```python
from build123d import *

# Parameters (mm, degrees)
SKETCH2_W           = 127
SKETCH2_H           = 70
BOSS_EXTRUDE1_DEPTH = 55
SKETCH4_W           = 127
SKETCH4_H           = 30
CUT_EXTRUDE1_DEPTH  = 50
SKETCH5_W           = 15
SKETCH5_H           = 23
BOSS_EXTRUDE2_DEPTH = 23
SKETCH6_W           = 3
SKETCH6_H           = 23
CUT_EXTRUDE2_DEPTH  = 23
SKETCH9_W           = 15
SKETCH9_H           = 10
CUT_EXTRUDE3_DEPTH  = 11.5
SKETCH10_W          = 117
SKETCH10_H          = 60
CUT_EXTRUDE4_DEPTH  = 1
SKETCH12_R          = 5
CUT_EXTRUDE5_DEPTH  = 300


with BuildPart() as part:
    # Sketch2 → Boss-Extrude1 (new body)
    with BuildSketch(Plane(origin=(0, 0, 0), x_dir=(1, 0, 0), z_dir=(0, 1, 0))):
        Rectangle(SKETCH2_W, SKETCH2_H)
    extrude(amount=BOSS_EXTRUDE1_DEPTH)

    # Sketch4 → Cut-Extrude1 (cut)
    with BuildSketch(Plane(origin=(0, 0, 0), x_dir=(1, 0, 0), z_dir=(0, 1, 0))):
        Rectangle(SKETCH4_W, SKETCH4_H)
    extrude(amount=CUT_EXTRUDE1_DEPTH, mode=Mode.SUBTRACT)

    # Sketch5 → Boss-Extrude2 (add)
    with BuildSketch(Plane.XZ.offset(-50)):
        Rectangle(SKETCH5_W, SKETCH5_H)
    extrude(amount=BOSS_EXTRUDE2_DEPTH)

    # Sketch6 → Cut-Extrude2 (cut)
    with BuildSketch(Plane.XZ.offset(-27)):
        with Locations((5, 0)):
            Rectangle(SKETCH6_W, SKETCH6_H)
    extrude(amount=-CUT_EXTRUDE2_DEPTH, mode=Mode.SUBTRACT)

    # Sketch9 → Cut-Extrude3 (cut)
    with BuildSketch(Plane(origin=(0, 27, 0), x_dir=(1, 0, 0), z_dir=(0, 1, 0))):
        Rectangle(SKETCH9_W, SKETCH9_H)
    extrude(amount=CUT_EXTRUDE3_DEPTH, mode=Mode.SUBTRACT)

    # Sketch10 → Cut-Extrude4 (cut)
    with BuildSketch(Plane(origin=(0, 55, 0), x_dir=(1, 0, 0), z_dir=(0, 1, 0))):
        Rectangle(SKETCH10_W, SKETCH10_H)
    extrude(amount=-CUT_EXTRUDE4_DEPTH, mode=Mode.SUBTRACT)

    # Sketch12 → Cut-Extrude5 (cut)
    with BuildSketch(Plane.ZY.offset(7.5)):
        with Locations((0, 38.5)):
            Circle(SKETCH12_R)
    extrude(amount=-CUT_EXTRUDE5_DEPTH, mode=Mode.SUBTRACT)


solid = part.part
```
Build history of the part. All positions in model axes, mm. A direction names the side the tool comes from. Round coordinates to 2 decimals unless told otherwise and drop trailing zeros. Write each loop counter-clockwise with the first axis right and the second up, starting at its lowest first coordinate (ties: lowest second). Pieces come first, ordered by that corner, then holes.
1) Band-saw the part on D-D, the plane z = 0. List the corners of the cut face in (x, y), and give its area (3 significant figures).
2) Drill centre lines: probe 1 along Z at (x, y) = (-15, 32); probe 2 along X at (y, z) = (44, -6.5); probe 3 along Y at (x, z) = (-28, 6). Where is each one in solid material? Low to high.
3) Band-saw the part on A-A, the plane y = 20. List the corners of the cut face in (x, z), and give its area (3 significant figures).
4) Band-saw the part on B-B, the plane x = 30.5. List the corners of the cut face in (y, z).
5) Band-saw the part on C-C, the plane z = 27. List the corners of the cut face in (x, y).
6) Pin check, flat tips, straight feed: pin 1 (1.5 mm diameter, centred on x = -36, z = 11.5, fed in from +Y); pin 2 (11.5 mm diameter, centred on y = 37, z = -3, fed in from +X); pin 3 (9 mm diameter, centred on x = 30, z = -7.5, fed in from -Y). Stop position of each tip, or through.
7) 3-axis set-ups, long thin cutter, end or side, ignore diameter. For faces 1 (the flat face through (63.5, 27, 16)), 2 (the flat face through (-2, 27, 8)), 3 (the flat face through (7.5, 44, 0)), 4 (the flat face through (-7.5, 44, 0)), 5 (the flat face through (-1, 54, 0)): which of +Z, -Z, +X, -X, +Y, -Y reach the whole face in a straight line?
8) Mould opens along Z. For faces 6 (the flat face through (-1, 0, 25)), 7 (the cylindrical face through (-2.1, 43.5, 0.1)), 8 (the flat face through (-1, 27, 35)), 9 (the flat face through (3.5, 43, -3)) say: +Z half, -Z half, draft (parallel to the pull), parting line (faces both ways), or undercut.
Ans:
1. outline: (-63.5, 50) - (-7.5, 50) - (-7.5, 43.5) - (3.5, 43.5) - (3.5, 50) - (6.5, 50) - (6.5, 43.5) - (7.5, 43.5) - (7.5, 50) - (63.5, 50) - (63.5, 55) - (58.5, 55) - (58.5, 54) - (-58.5, 54) - (-58.5, 55) - (-63.5, 55) - close
1. area: 596 mm2
2. probe 1: z = -35 to -15, 15 to 35
2. probe 2: x = -7.5 to 3.5, 6.5 to 7.5
2. probe 3: y = 50 to 54
3. outline: (-63.5, -35) - (63.5, -35) - (63.5, -15) - (-63.5, -15) - close; (-63.5, 15) - (63.5, 15) - (63.5, 35) - (-63.5, 35) - close
3. area: 5,080 mm2
4. outline: (0, -35) - (55, -35) - (55, -30) - (54, -30) - (54, 30) - (55, 30) - (55, 35) - (0, 35) - (0, 15) - (50, 15) - (50, -15) - (0, -15) - close
5. outline: (-63.5, 0) - (63.5, 0) - (63.5, 55) - (58.5, 55) - (58.5, 54) - (-58.5, 54) - (-58.5, 55) - (-63.5, 55) - close
6. pin 1: stops at y = 54
6. pin 2: stops at x = 7.5
6. pin 3: stops at y = 50
7. face 1: +Z, -Z, +X, +Y, -Y
7. face 2: +X, -X, -Y
7. face 3: +X, -Y
7. face 4: -X, -Y
7. face 5: +Y
8. face 6: draft
8. face 7: undercut
8. face 8: +Z half
8. face 9: undercut
